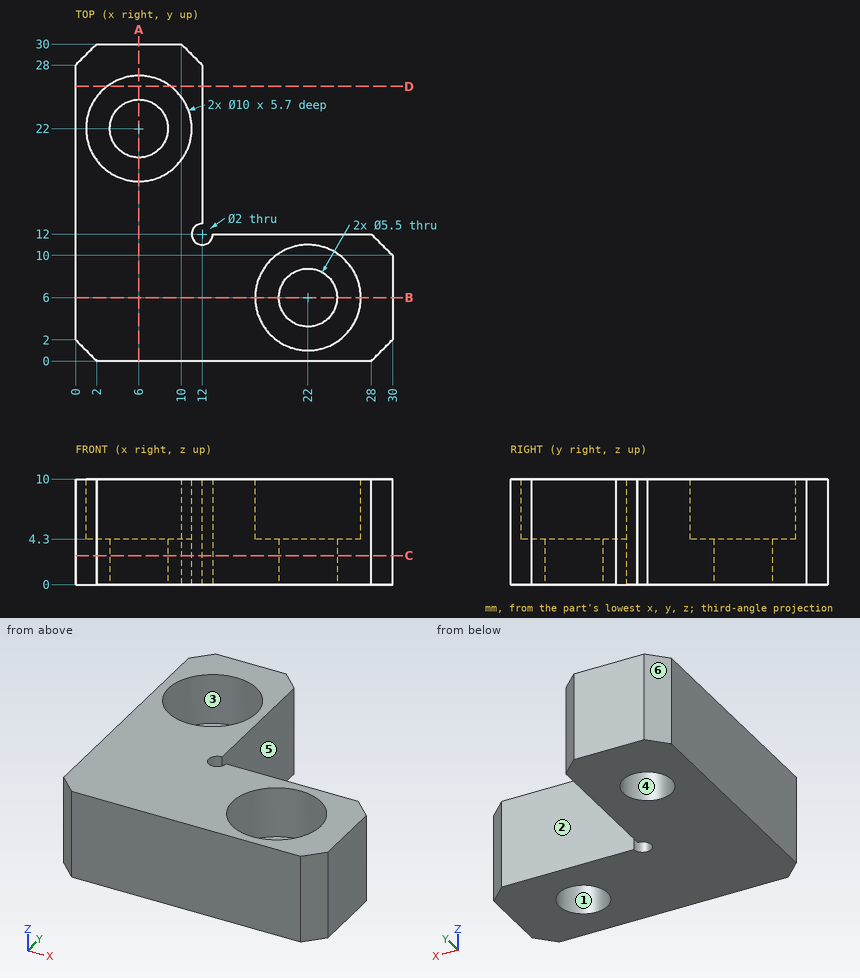
Design review of the part shown in the three views and the two pictorial views. Dimensions are in mm from the part's minimum x, y and z. A direction names the side the tool comes from. Round coordinates to 2 decimals unless told otherwise and drop trailing zeros. Loops run counter-clockwise (first coordinate to the right, second up) from the corner with the lowest first, then second, coordinate; pieces in that order, holes last. Notation, with made-up numbers: (49.25, 19) - (100.25, 19) arc R31 ccw to (100.25, 43) - close; hole circle Ø8 at (-31.5, 3.5). An arc over 180 degrees is marked (long way). Write each question's results on one line, items separated by ' | '. Start each with the question number.
Q1. Wall thickness on line 1 along Y through (x, z) = (6, 7.1); line 2 along Y through (x, z) = (6, 1.8); line 3 along X through (y, z) = (8.5, 9.25): over which ranges is each line inside the solid? List them lowest first. Write a range as [from, to].
Q2. Insertion check: P1, Ø5, axis at x = 6, y = 22, coming from the +Z side; P2, Ø2.5, axis at x = 12, y = 12, coming from the -Z side; P3, Ø3, axis at x = 4.5, y = 23.5, coming from the +Z side; P4, Ø5, axis at y = 20, z = 5.5, coming from the +X side. Each pin has a flat end and moves straight along its axis. Give the tip position at first contact, or say it passes through.
Q3. Take a section at D-D on y = 26. Give the boundary of the cut face in (x, z), plus the area to 3 significant figures.
Q4. Draft analysis for pull direction X (two halves, no side actions). For the marked faces 4, 5 and 6, state which applies: pulls with the +X half, pulls with the -X half, needs draft (parallel to the pull), parting line crosses it, or undercut.
Q5. Take a section at A-A on x = 6. Give the boundary of the cut face in (y, z), plus the area to 3 significant figures.
Q6. Take a section at C-C on z = 2.75. Give the boundary of the cut face in (x, y), plus the area to 3 significant figures.
Q7. Tool access review of the marked faces 1, 2 and 3: name each direction out of +Z, -Z, +X, -X, +Y, -Y from which nothing blocks a thin tool from reaching the whole face with its end or side.
Data:
1) line 1: y = [0, 17], [27, 30] | line 2: y = [0, 19.25], [24.75, 30] | line 3: x = [0, 17.67], [26.33, 30]
2) P1: passes through | P2: stops at z = 0 | P3: stops at z = 4.3 | P4: stops at x = 12
3) outline: (0, 0) - (12, 0) - (12, 10) - (9, 10) - (9, 4.3) - (3, 4.3) - (3, 10) - (0, 10) - close | area: 85.8 mm²
4) face 4: undercut | face 5: pulls with the +X half | face 6: pulls with the -X half
5) outline: (0, 0) - (19.25, 0) - (19.25, 4.3) - (17, 4.3) - (17, 10) - (0, 10) - close; (24.75, 0) - (30, 0) - (30, 10) - (27, 10) - (27, 4.3) - (24.75, 4.3) - close | area: 219 mm²
6) outline: (0, 2) - (2, 0) - (28, 0) - (30, 2) - (30, 10) - (28, 12) - (13, 12) arc R1 cw (long way) to (12, 13) - (12, 28) - (10, 30) - (2, 30) - (0, 28) - close; hole circle Ø5.5 at (6, 22); hole circle Ø5.5 at (22, 6) | area: 516 mm²
7) face 1: +Z, -Z | face 2: +Z, -Z, +X, +Y | face 3: +Z
